Could you check a few things on this model? Use its own coordinates, in mm. A direction names the side the tool comes from. Give positions to 0.01 mm unless a question says otherwise; leave off trailing zeros. Write each loop counter-clockwise with the first axis right and the second up, starting at its lowest first coordinate (ties: lowest second). Pieces come first, ordered by that corner, then holes. Notation, with made-up numbers: (48, 62.25) -> (62, 62.25) arc R25 cw to (62, 78.25) -> close; hole circle Ø5 at (-30, -30). An arc over 180 degrees is marked (long way). One line per question, with ' | ' between items.
Autodesk Inventor part; units mm, degrees
ref_plane "Work Plane1" through (0, 12.5, 0) normal (0, 1, 0) x (-1, 0, 0)
ref_plane "YZ Plane" through (0, 0, 0) normal (1, 0, 0) x (0, 1, 0)
ref_plane "XY Plane" through (0, 0, 0) normal (0, 0, 1) x (1, 0, 0)
sketch "Sketch1" plane through (0, 0, 0) normal (0, 0, 1) x (1, 0, 0)
  circle A0 centre (0, 0) radius 6
  circle A1 centre (0, 0) radius 12.5
  dimension "d0" = 12
  dimension "d1" = 25
extrude "Extrusion1" add sketch "Sketch1" along normal blind 10
sketch "Sketch2" plane through (0, 0, 0) normal (0, 1, 0) x (-1, 0, 0)
  circle A0 centre (0, 5) radius 2.5
  line L0 (6, 0) -> (6, 10)
  point P0 (0, 0)
  point P1 (6, 5)
  dimension "d4" = 5
extrude "Extrusion2" cut sketch "Sketch2" along normal through all both and the other way through all
ref_plane "Work Plane1" through (0, 12.5, 0) normal (0, 1, 0) x (-1, 0, 0)
sketch "Sketch4" plane through (0, 12.5, 0) normal (0, 1, 0) x (-1, 0, 0)
  spline S0 degree 8 poles (2.5, 5) (2.5, 5.2613) (2.4688, 5.5221) (2.4066, 5.7804) (2.3127, 6.0339) (2.1861, 6.2798) (2.0251, 6.5144) (1.828, 6.7323) (1.3947, 7.0908) (1.1606, 7.2449) (0.8947, 7.3748) (0.6036, 7.4701) (0.2962, 7.5238) (-0.0173, 7.5328) (-0.3265, 7.4973) (-0.927, 7.3431) (-1.2062, 7.2245) (-1.4564, 7.0744) (-1.6765, 6.9) (-1.8664, 6.7071) (-2.0266, 6.5008) (-2.1581, 6.2854) (-2.3815, 5.8106) (-2.4663, 5.546) (-2.5169, 5.2746) (-2.5338, 5) (-2.5169, 4.7254) (-2.4663, 4.454) (-2.3815, 4.1894) (-2.1645, 3.7282) (-2.0429, 3.5262) (-1.8964, 3.3322) (-1.7241, 3.1495) (-1.5253, 2.9819) (-1.3, 2.8342) (-1.0485, 2.712) (-0.5121, 2.5377) (-0.2336, 2.4833) (0.0549, 2.4652) (0.3445, 2.486) (0.6257, 2.5448) (0.8897, 2.6372) (1.1293, 2.7558) (1.6409, 3.0804) (1.8944, 3.3103) (2.1007, 3.5658) (2.2623, 3.8384) (2.3815, 4.1219) (2.4604, 4.412) (2.5, 4.7056) (2.5, 5) knots 0 0 0 0 0 0 0 0 0 0.155158 0.155158 0.155158 0.155158 0.155158 0.155158 0.155158 0.286737 0.286737 0.286737 0.286737 0.286737 0.286737 0.286737 0.422792 0.422792 0.422792 0.422792 0.422792 0.422792 0.422792 0.579084 0.579084 0.579084 0.579084 0.579084 0.579084 0.579084 0.706752 0.706752 0.706752 0.706752 0.706752 0.706752 0.706752 0.82726 0.82726 0.82726 0.82726 0.82726 0.82726 0.82726 1 1 1 1 1 1 1 1 1
  circle A0 centre (0, 5) radius 6.5
  point P0 (0, 0)
  dimension "d8" = 13
extrude "Extrusion3" cut sketch "Sketch4" against normal blind 5
properties part number "WA003.ip" material "ABS Plastic"
Q1. Will these pins go through, and if not, where does the flat tip stop? pin 1 (5 mm diameter, centred on x = 1.5, z = 6, fed in from +Y); pin 2 (4 mm diameter, centred on y = 8.5, z = 8, fed in from +X); pin 3 (1.5 mm diameter, centred on x = 9, z = 5.5, fed in from -Y); pin 4 (4 mm diameter, centred on x = 0, z = 5, fed in from -Y).
Answer below:
pin 1: stops at y = 7.5 | pin 2: stops at x = 10.68 | pin 3: stops at y = -9.39 | pin 4: passes through
Q2. If I drill on line 1 along Z through (x, y) = (0, -8); line 2 along Y through (x, z) = (0, 9.75); line 3 along X through (y, z) = (-5.5, 5.25), over which ranges is the centre line in solid material (lowest first)?
Answer below:
line 1: z = 0 to 2.5, 7.5 to 10 | line 2: y = -12.5 to -6, 6 to 7.5 | line 3: x = -11.22 to -2.49, 2.49 to 11.22
Q3. Imagine slicing it at C-C on z = 5. Please give me the cut outline in (x, y), and give its area (3 significant figures).
Answer below:
outline: (-6.5, 7.5) -> (-6.5, 10.68) arc R12.5 ccw to (-2.5, -12.25) -> (-2.5, -5.45) arc R6 cw to (-2.5, 5.45) -> (-2.5, 7.5) -> close; (2.5, -12.25) arc R12.5 ccw to (6.5, 10.68) -> (6.5, 7.5) -> (2.5, 7.5) -> (2.5, 5.45) arc R6 cw to (2.5, -5.45) -> close | area: 279 mm^2
Q4. Imagine slicing it at A-A on y = 0. Please give me the cut outline in (x, z).
Answer below:
outline: (-12.5, 0) -> (-6, 0) -> (-6, 10) -> (-12.5, 10) -> close; (6, 0) -> (12.5, 0) -> (12.5, 10) -> (6, 10) -> close
Q5. Imagine slicing it at D-D on x = -5.5. Please give me the cut outline in (y, z), and give its area (3 significant figures).
Answer below:
outline: (-11.22, 0) -> (-2.4, 0) -> (-2.4, 10) -> (-11.22, 10) -> close; (2.4, 0) -> (11.22, 0) -> (11.22, 1.54) -> (7.5, 1.54) -> (7.5, 8.46) -> (11.22, 8.46) -> (11.22, 10) -> (2.4, 10) -> close | area: 151 mm^2
Q6. Imagine slicing it at B-B on x = 0. Please give me the cut outline in (y, z).
Answer below:
outline: (-12.5, 0) -> (-6, 0) -> (-6, 2.5) -> (-12.5, 2.5) -> close; (-12.5, 7.5) -> (-6, 7.5) -> (-6, 10) -> (-12.5, 10) -> close; (6, 0) -> (7.5, 0) -> (7.5, 2.5) -> (6, 2.5) -> close; (6, 7.5) -> (7.5, 7.5) -> (7.5, 10) -> (6, 10) -> close
Q7. If we mould it in two halves opening along Y, with no side actions, what happens to faces 3 (the cylindrical face through (2.769, 5.323, 4.93)), 4 (the cylindrical face through (2.5, -8.9, 5.1)), 5 (the flat face through (2, 7.5, 7))? For each: +Y half, -Y half, draft (parallel to the pull), parting line (faces both ways), or undercut.
Answer below:
face 3: undercut | face 4: draft | face 5: +Y half
Q8. On a 3-axis mill with a long thin cutter (end or side, diameter ignored), from which of +Z, -Z, +X, -X, +Y, -Y can I reach the whole of each face in a straight line? I mean faces 1 (the flat face through (3, -6, 0)), 2 (the cylindrical face through (6.5, 9.2, 5.1)). Say none if no direction works.
Answer below:
face 1: -Z, +X, -X, +Y, -Y | face 2: +Y
